Check sheet for the drawn part. Datum: minimum x, y, z corner. Units: mm. A direction names the side the tool comes from. Coordinates: 2 decimals unless noted, no trailing zeros. Write each loop counter-clockwise with the first axis right and the second up, starting at its lowest first coordinate (ties: lowest second). Pieces come first, ordered by that corner, then holes. Notation, with made-up numbers: (82.5, 75.25) -> (105.5, 75.25) arc R18 cw to (105.5, 91.25) -> close; hole circle Ø3 at (27.5, 10). An arc over 180 degrees is marked (long way). One line per question, with ' | ' between items.
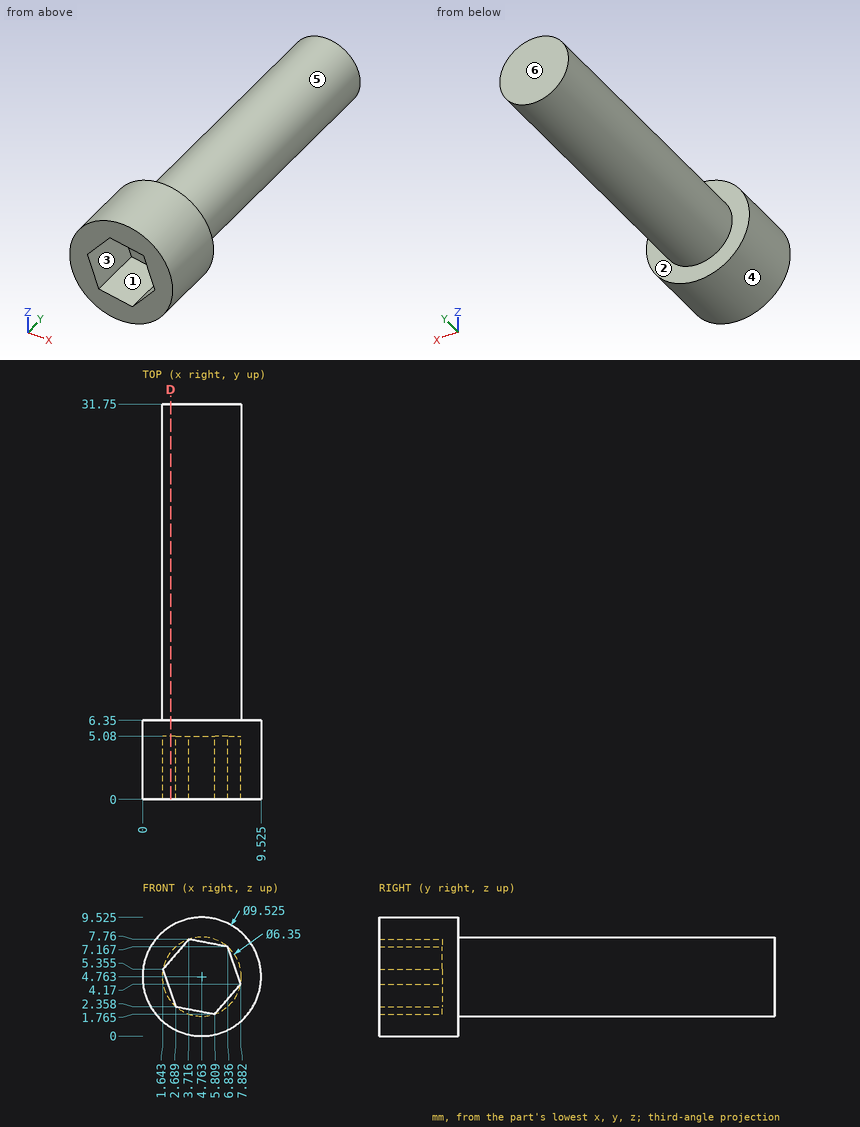
1. Mould release check, pull along X, two halves, no side actions. Record for the marked faces 1, 2, 3 and 4: released by +X, released by -X, zero draft, split by the parting line, or undercut.
Worked answers:
face 1: undercut | face 2: zero draft | face 3: undercut | face 4: split by the parting line
2. Tool access check on the marked faces 5 and 6. Record the directions out of +Z, -Z, +X, -X, +Y, -Y that give a thin tool (end or side, any length) a straight path to the whole face; none if there is none.
Worked answers:
face 5: +Y | face 6: +Z, -Z, +X, -X, +Y
3. Go/stop test with flat-tipped pins: P1, Ø1, axis at x = 2.5, y = 7, coming from the -Z side; P2, Ø3, axis at x = 4.5, z = 4, coming from the -Y side; P3, Ø4, axis at y = 22, z = 5.5, coming from the +X side. Record where each tip stops, or that it passes through.
Worked answers:
P1: z = 2.12 | P2: y = 5.08 | P3: x = 7.94
4. Cross-section at D-D on x = 2.25. Record the boundary of the cut face in (y, z).
Worked answers:
outline: (0, 0.72) -> (6.35, 0.72) -> (6.35, 2.82) -> (31.75, 2.82) -> (31.75, 6.7) -> (6.35, 6.7) -> (6.35, 8.81) -> (0, 8.81) -> (0, 6.06) -> (5.08, 6.06) -> (5.08, 3.62) -> (0, 3.62) -> close
5. Material ranges on line 1 (Y direction, x = 7.25, z = 5); line 2 (Y direction, x = 4, z = 8.75); line 3 (Z direction, x = 4.5, y = 6), recorded low to high. Write a range as from..to.
Worked answers:
line 1: 5.08..31.75 | line 2: 0..6.35 | line 3: 0.01..9.52
